```python
from build123d import *

# Parameters (mm, degrees)
SKETCH1_R           = 20.000000005
BOSS_EXTRUDE1_DEPTH = 6.35
BOSS_EXTRUDE2_DEPTH = 3.175
SKETCH3_R           = 1.5875
CUT_EXTRUDE1_DEPTH  = 30.525000005
CUT_EXTRUDE2_DEPTH  = 3.175


with BuildPart() as part:
    # Sketch1 → Boss-Extrude1 (new body)
    with BuildSketch(Plane(origin=(0, 0, 0), x_dir=(1, 0, 0), z_dir=(0, 1, 0))):
        Circle(SKETCH1_R)
    extrude(amount=BOSS_EXTRUDE1_DEPTH)

    # Sketch2 → Boss-Extrude2 (add)
    with BuildSketch(Plane(origin=(6.35, 0, 0), x_dir=(0, 0, -1), z_dir=(1, 0, 0))):
        with BuildLine():
            Line((-17.420082718, 0), (-17.420082718, -4.254))
            ThreePointArc((-17.420082718, -4.254), (-14.245082718, -7.429), (-11.070082718, -4.254))
            Line((-11.070082718, -4.254), (-11.070082718, -3.175))
            ThreePointArc((-11.070082718, -3.175), (-10.140146748, -0.92993597), (-7.895082718, 0))
            Line((-7.895082718, 0), (-5.849160659, 0))
            Line((-5.849160659, 0), (-5.849160659, 6.35))
            Line((-5.849160659, 6.35), (-11.070082718, 6.35))
            ThreePointArc((-11.070082718, 6.35), (-15.560210778, 4.490128061), (-17.420082718, 0))
        make_face()
    boss_extrude2 = extrude(amount=BOSS_EXTRUDE2_DEPTH)

    # Mirror1: Boss-Extrude2 across plane
    add(boss_extrude2.mirror(Plane(origin=(0, 0, 0), x_dir=(0, 0, 1), z_dir=(1, 0, 0))))

    # Sketch3 → Cut-Extrude1 (cut, through all)
    with BuildSketch(Plane(origin=(9.525, 0, 0), x_dir=(0, 0, -1), z_dir=(1, 0, 0))):
        with Locations((-14.245082718, -4.254)):
            Circle(SKETCH3_R)
    extrude(amount=-CUT_EXTRUDE1_DEPTH, mode=Mode.SUBTRACT)

    # Sketch5 → Cut-Extrude2 (cut)
    with BuildSketch(Plane.XZ):
        with BuildLine():
            Line((6.35, 18.965165441), (6.35, 7.605609073))
            ThreePointArc((6.35, 7.605609073), (0, -9.907965955), (-6.35, 7.605609073))
            Line((-6.35, 7.605609073), (-6.35, 18.965165441))
            ThreePointArc((-6.35, 18.965165441), (0, 20.000000005), (6.35, 18.965165441))
        make_face()
    extrude(amount=-CUT_EXTRUDE2_DEPTH, mode=Mode.SUBTRACT)


solid = part.part
```
Input: part model. Units: mm. Frame: model coordinates. A direction names the side the tool comes from. Give positions to 0.01 mm unless a question says otherwise; leave off trailing zeros. Order: outer loops, then holes, each group sorted by start corner. A loop starts at its lowest first (then second) coordinate and runs counter-clockwise, first axis right, second up. Notation, with made-up numbers: M -4,4.25 L 41,4.25 A14 ccw 41,21.25 Z; hole C -12,50 d9. An arc over 180 degrees is marked long. Return JSON: item names as keys, results as strings.
Item 1: Ray query, probe 1 along X at (y, z) = (2.3, 0); probe 2 along Y at (x, z) = (12.5, 4); probe 3 along Y at (x, z) = (3, 11) (3 decimals). Return the intervals inside material, ascending.
Solutions:
{"probe 1": "-20 to -9.91, 9.91 to 20", "probe 2": "0 to 6.35", "probe 3": "3.175 to 6.35"}
Item 2: Cut plane C-C (x = 0). Return loops of the section in (y, z) (3 decimals).
Solutions:
{"outline": "M 0,-20 L 6.35,-20 L 6.35,20 L 3.175,20 L 3.175,-9.908 L 0,-9.908 Z"}
Item 3: Cut plane B-B (y = -2). Return loops of the section in (x, z) (3 decimals).
Solutions:
{"outline": "M -9.525,10.845 L -6.35,10.845 L -6.35,17.42 L -9.525,17.42 Z; M 6.35,10.845 L 9.525,10.845 L 9.525,17.42 L 6.35,17.42 Z"}
Item 4: First-contact query: P1, Ø22, axis at x = 2.5, z = -2, coming from the -Y side; P2, Ø1.6, axis at x = 8, y = -2, coming from the +Z side; P3, Ø1, axis at x = 7.5, y = -5.5, coming from the -Z side; P4, Ø1.5, axis at x = 0, y = -2, coming from the -Z side. Flat tips, straight axial feed; report the tip coordinate or a pass-through.
Solutions:
{"P1": "y = -0.03", "P2": "z = 17.42", "P3": "z = 11.16", "P4": "through"}
Item 5: Access query for faces 1 (the flat face through (6.35, -1, 13)), 2 (the flat face through (-8, -2, 17.42)), 3 (the flat face through (9.525, -2, 14)), 4 (the flat face through (8, -4, 11.07)). Directions: +Z, -Z, +X, -X, +Y, -Y. A direction counts if a zero-diameter tool reaches every point of the face in a straight line with its end or side. Return the directions, or none.
Solutions:
{"face 1": "+Z, -Y", "face 2": "+Z, +X, -X, -Y", "face 3": "+Z, -Z, +X, -Y", "face 4": "-Z, +X, -X, -Y"}
Item 6: Pull-direction query (Y, two-part tool) for faces 5 (the cylindrical face through (0.339, 1.565, -9.902)), 6 (the cylindrical face through (7.92, -7.43, 14.31)), 7 (the cylindrical face through (-7.92, -3.78, 12.73)); classes: +Y half, -Y half, draft (parallel to the pull), parting line (faces both ways), or undercut.
Solutions:
{"face 5": "draft", "face 6": "-Y half", "face 7": "undercut"}
Item 7: Cut plane D-D (y = 5). Return loops of the section in (x, z), then the cut area to 3 significant figures.
Solutions:
{"outline": "C 0,0 d40", "area": "1,260 mm^2"}
Item 8: Cut plane A-A (z = 0). Return loops of the section in (x, y) (3 decimals).
Solutions:
{"outline": "M -20,0 L -9.908,0 L -9.908,3.175 L 9.908,3.175 L 9.908,0 L 20,0 L 20,6.35 L -20,6.35 Z"}
